The model under review builds one solid part; all positions refer to its coordinate system, in mm. Round coordinates to 2 decimals unless told otherwise and drop trailing zeros. Loops run counter-clockwise (first coordinate to the right, second up) from the corner with the lowest first, then second, coordinate; pieces in that order, holes last. Notation, with made-up numbers: (46, 38) -> (52, 38) arc R23 ccw to (52, 69) -> close; hole circle Ø9 at (-31.5, 30.5). An arc over 180 degrees is marked (long way). Write each question's results on one line, items separated by ' | '. Start each with the question number.
Item 1: For L1, parallel to Y at x = 23.5, z = 2.9; L2, parallel to X at y = 36, z = 2.15; L3, parallel to X at y = 38.5, z = 2.25, list the stretches that pass through material, from the lowest coordinate up. Write a range as from..to.
Item 2: We need section B-B (z = 0.9). Give the number of separate pieces and of enclosed holes in the cut face, and give its area (3 significant figures).
Item 3: We need section C-C (x = 49). Give the boundary of the cut face in (y, z), and give its area (3 significant figures).
Item 4: We need section A-A (x = 33). Give the boundary of the cut face in (y, z), and give its area (3 significant figures).
Item 5: Clearance check with flat-ended pins moving along their axes: pin 1 Ø1.5 at (y, z) = (11, 2) entering from -X; pin 2 Ø1.5 at (y, z) = (38.5, 1) entering from +X; pin 3 Ø2.5 at (x, y) = (26.12, 12.58) entering from +Z; pin 4 Ø0.9 at (y, z) = (10, 1) entering from -X. State where each tip first meets the part, or that it passes through.
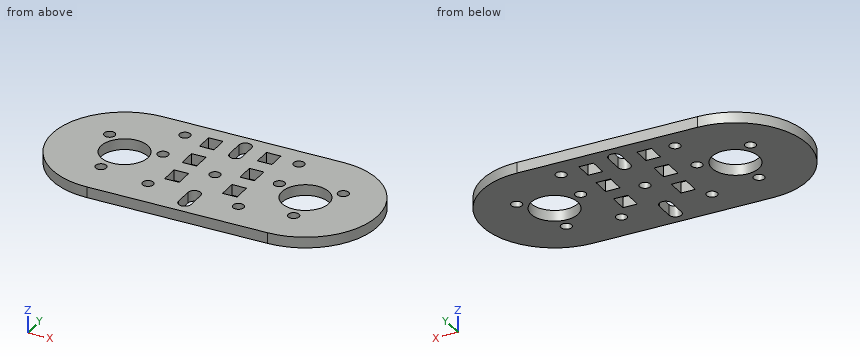
from build123d import *

# Parameters (mm, degrees)
SKETCH_1_R      = 1.5
SKETCH_1_R_2    = 6.5
SKETCH_1_W      = 4
SKETCH_1_H      = 4.8
SKETCH_1_H_2    = 5
EXTRUDE_1_DEPTH = 3


with BuildPart() as part:
    # 草图1 → 凸台-拉伸1 (new body)
    with BuildSketch(Plane.XY):
        with BuildLine():
            Line((38.62258193, 44.104762576), (19.62258193, 44.104762576))
            Line((19.62258193, 44.104762576), (17.62258193, 44.104762576))
            Line((17.62258193, 44.104762576), (9.62258193, 44.104762576))
            Line((9.62258193, 44.104762576), (7.62258193, 44.104762576))
            Line((7.62258193, 44.104762576), (-11.37741807, 44.104762576))
            ThreePointArc((-11.37741807, 44.104762576), (-31.37741807, 24.104762576), (-11.37741807, 4.104762576))
            Line((-11.37741807, 4.104762576), (38.62258193, 4.104762576))
            ThreePointArc((38.62258193, 4.104762576), (58.62258193, 24.104762576), (38.62258193, 44.104762576))
        make_face()
        with Locations((29.703887727, 27.376901588)):
            Circle(SKETCH_1_R, mode=Mode.SUBTRACT)
        with Locations((-2.458723867, 27.376901588)):
            Circle(SKETCH_1_R, mode=Mode.SUBTRACT)
        with Locations((-13.003009663, 14.744877322)):
            Circle(SKETCH_1_R, mode=Mode.SUBTRACT)
        with Locations((-18.670520681, 30.192508819)):
            Circle(SKETCH_1_R, mode=Mode.SUBTRACT)
        with Locations((45.91568454, 30.192508819)):
            Circle(SKETCH_1_R, mode=Mode.SUBTRACT)
        with Locations((-11.37741807, 24.104762576)):
            Circle(SKETCH_1_R_2, mode=Mode.SUBTRACT)
        with Locations((38.62258193, 24.104762576)):
            Circle(SKETCH_1_R_2, mode=Mode.SUBTRACT)
        with Locations((29.363598717, 38.36208455)):
            Circle(SKETCH_1_R, mode=Mode.SUBTRACT)
        with Locations((13.62258193, 24.104762576)):
            Circle(SKETCH_1_R, mode=Mode.SUBTRACT)
        with Locations((-2.118434858, 38.36208455)):
            Circle(SKETCH_1_R, mode=Mode.SUBTRACT)
        with Locations((40.248173522, 14.744877322)):
            Circle(SKETCH_1_R, mode=Mode.SUBTRACT)
        with Locations((26.12258193, 12.583043954)):
            Circle(SKETCH_1_R, mode=Mode.SUBTRACT)
        with Locations(Location((1.12258193, 12.583043954, 0), (0, 0, 180))):
            Circle(SKETCH_1_R, mode=Mode.SUBTRACT)
        with Locations((21.62258193, 37.474762576)):
            Rectangle(SKETCH_1_W, SKETCH_1_H, mode=Mode.SUBTRACT)
        with Locations((21.62258193, 28.344762576)):
            Rectangle(SKETCH_1_W, SKETCH_1_H_2, mode=Mode.SUBTRACT)
        with Locations((5.62258193, 37.474762576)):
            Rectangle(SKETCH_1_W, SKETCH_1_H, mode=Mode.SUBTRACT)
        with Locations((5.62258193, 28.344762576)):
            Rectangle(SKETCH_1_W, SKETCH_1_H_2, mode=Mode.SUBTRACT)
        with Locations((5.62258193, 19.114762576)):
            Rectangle(SKETCH_1_W, SKETCH_1_H_2, mode=Mode.SUBTRACT)
        with Locations((21.62258193, 19.114762576)):
            Rectangle(SKETCH_1_W, SKETCH_1_H_2, mode=Mode.SUBTRACT)
        with BuildLine():
            Line((11.87258193, 8.127075217), (11.87258193, 13.127075217))
            ThreePointArc((11.87258193, 13.127075217), (13.62258193, 14.877075217), (15.37258193, 13.127075217))
            Line((15.37258193, 13.127075217), (15.37258193, 8.127075217))
            ThreePointArc((15.37258193, 8.127075217), (13.62258193, 6.377075217), (11.87258193, 8.127075217))
        make_face(mode=Mode.SUBTRACT)
        with BuildLine():
            Line((15.37258193, 40.127075217), (15.37258193, 35.127075217))
            ThreePointArc((15.37258193, 35.127075217), (13.62258193, 33.377075217), (11.87258193, 35.127075217))
            Line((11.87258193, 35.127075217), (11.87258193, 40.127075217))
            ThreePointArc((11.87258193, 40.127075217), (13.62258193, 41.877075217), (15.37258193, 40.127075217))
        make_face(mode=Mode.SUBTRACT)
    extrude(amount=EXTRUDE_1_DEPTH)


solid = part.part
Here are the results:
1) L1: y = 4.1..16.61, 21.61..25.84, 30.84..35.07, 39.87..44.1 | L2: x = -27.46..3.62, 7.62..11.87, 15.37..19.62, 23.62..54.7 | L3: x = -25.26..-3.61, -0.62..3.62, 7.62..11.87, 15.37..19.62, 23.62..27.87, 30.86..52.51
2) separate pieces: 1 | enclosed holes: 21 | area: 2,740 mm2
3) outline: (7.01, 0) -> (41.2, 0) -> (41.2, 3) -> (7.01, 3) -> close | area: 103 mm2
4) outline: (4.1, 0) -> (20.84, 0) -> (20.84, 3) -> (4.1, 3) -> close; (27.37, 0) -> (44.1, 0) -> (44.1, 3) -> (27.37, 3) -> close | area: 100 mm2
5) pin 1: stops at x = -27.11 | pin 2: stops at x = 53.24 | pin 3: passes through | pin 4: stops at x = -25.99
